from build123d import *

# Parameters (mm, degrees)
CUT_EXTRUDE1_DEPTH = 0.8


with BuildPart() as part:
    # Sketch2 → Revolve1 (revolve)
    with BuildSketch(Plane.XY):
        with BuildLine():
            Line((0, 0), (0, 1.8))
            ThreePointArc((0, 1.8), (0.058578644, 1.941421356), (0.2, 2))
            Line((0.2, 2), (1.8, 2))
            ThreePointArc((1.8, 2), (1.941421356, 1.941421356), (2, 1.8))
            Line((2, 1.8), (2, 1))
            Line((2, 1), (6.75, 1))
            Line((6.75, 1), (7, 0.75))
            Line((7, 0.75), (7, 0))
            Line((7, 0), (0, 0))
        make_face()
    revolve(axis=Axis((-2.281841559, 0, 0), (1, 0, 0)))

    # Sketch3 → Cut-Extrude1 (cut)
    with BuildSketch(Plane.ZY):
        Polygon((0.433012702, -0.75), (0.866025404, 0), (0.433012702, 0.75), (-0.433012702, 0.75), (-0.866025404, 0), (-0.433012702, -0.75), align=None)
    extrude(amount=-CUT_EXTRUDE1_DEPTH, mode=Mode.SUBTRACT)


solid = part.part
Design review of the part built by this model. Coordinates are the model's own, in mm. A direction names the side the tool comes from. Round coordinates to 2 decimals unless told otherwise and drop trailing zeros. Write each loop counter-clockwise with the first axis right and the second up, starting at its lowest first coordinate (ties: lowest second). Pieces come first, ordered by that corner, then holes. Notation, with made-up numbers: (-21.75, 43) -> (2.25, 43) arc R32 ccw to (2.25, 69) -> close; hole circle Ø6 at (58, -8). An arc over 180 degrees is marked (long way). One line per item, written item: value. Start each with the question number.
Q1. Insertion check: P1, Ø2, axis at x = 5, z = -1.5, coming from the -Y side; P2, Ø1.5, axis at x = 4, z = -0.5, coming from the -Y side. Each pin has a flat end and moves straight along its axis. Give the tip position at first contact, or say it passes through.
Q2. The part is to be moulded in two halves that separate along Z. For faces 3 (the face through (0.8, 0, 0)), 4 (the face through (1, 0, -2)), 5 (the face through (7, 0, 0)), say which applies: pulls with the +Z half, pulls with the -Z half, needs draft (parallel to the pull), parting line crosses it, or undercut.
Q3. Add section B-B (x = 3). Give the boundary of the cut face in (y, z), then the cut area to 3 significant figures.
Q4. Tool access review of faces 1 (the face through (2, 1, -1)), 2 (the face through (0, -1, 0)): name each direction out of +Z, -Z, +X, -X, +Y, -Y from which nothing blocks a thin tool from reaching the whole face with its end or side.
Q5. To check wall thickness, follow probe 1 along Z at (x, y) = (2.25, 0.05); probe 2 along X at (y, z) = (-1.5, 0.45); probe 3 along X at (y, z) = (0.7, 0.05). State the ranges of each line that lie inside material, in increasing order.
Q6. Add section A-A (z = 0). Give the boundary of the cut face in (x, y).
Response:
1. P1: stops at y = -0.87
1. P2: stops at y = -1
2. face 3: undercut
2. face 4: parting line crosses it
2. face 5: needs draft
3. outline: circle Ø2 at (0, 0)
3. area: 3.14 mm^2
4. face 1: +X
4. face 2: +Z, -Z, -X, +Y, -Y
5. probe 1: z = -1 to 1
5. probe 2: x = 0 to 2
5. probe 3: x = 0.8 to 7
6. outline: (0, -1.8) arc R0.2 ccw to (0.2, -2) -> (1.8, -2) arc R0.2 ccw to (2, -1.8) -> (2, -1) -> (6.75, -1) -> (7, -0.75) -> (7, 0.75) -> (6.75, 1) -> (2, 1) -> (2, 1.8) arc R0.2 ccw to (1.8, 2) -> (0.2, 2) arc R0.2 ccw to (0, 1.8) -> (0, 0.75) -> (0.8, 0.75) -> (0.8, -0.75) -> (0, -0.75) -> close
